```python
from build123d import *

# Parameters (mm, degrees)
F0_R     = 7.5
F0_R_2   = 6.1
F1_DEPTH = 40
F2_R     = 1.6
F3_DEPTH = 1


with BuildPart() as f1:
    # F0 (on Front) → F1 (new body)
    with BuildSketch(Plane.XZ):
        Circle(F0_R)
        Circle(F0_R_2, mode=Mode.SUBTRACT)
    extrude(amount=F1_DEPTH)

    # F2 (on Top) → F3 (join, symmetric)
    with BuildSketch(Plane.XY):
        Polygon((14.5, 0), (6.5, 0), (6.5, -15.75), (14.5, -7.75), align=None)
        with Locations((11.25, -4.75)):
            Circle(F2_R, mode=Mode.SUBTRACT)
        Polygon((6.5, -24.25), (6.5, -40), (14.5, -40), (14.5, -32.25), align=None)
        with Locations((11.25, -35.25)):
            Circle(F2_R, mode=Mode.SUBTRACT)
        Polygon((-6.5, -33), (-6.5, -7), (-14.5, -18.25), (-14.5, -21.75), align=None)
        with Locations((-11.25, -20)):
            Circle(F2_R, mode=Mode.SUBTRACT)
    extrude(amount=F3_DEPTH, both=True)


solid = f1.part
```
CAD build for the part. Positions are in the model's coordinates, mm. A direction names the side the tool comes from. Round coordinates to 2 decimals unless told otherwise and drop trailing zeros. Loops run counter-clockwise (first coordinate to the right, second up) from the corner with the lowest first, then second, coordinate; pieces in that order, holes last. Notation, with made-up numbers: (80.25, -6.75) - (95.25, -6.75) arc R16 cw to (95.25, -2.75) - close; hole circle Ø9 at (-14, 26.5). An arc over 180 degrees is marked (long way). Return JSON: item names as keys, results as strings. Group by question number.
Q1. Two-plate mould, pull along X, no slides. Class faces 1 (the face through (9.65, -4.68, -0.01)), 2 (the face through (-11.016, -26.649, 0.014)), 3 (the face through (9, -6, -1)), 4 (the face through (14.5, -4, 0)): +X half, -X half, draft (parallel to the pull), parting line (faces both ways), or undercut.
Q2. Band-saw the part on A-A on x = 0. Give the cut face in (y, z).
Q3. Band-saw the part on C-C on z = 0. Give the cut face in (x, y), plus the area to 3 significant figures.
Q4. Flat gauge pins, fed straight in: pin 1 Ø4 at (y, z) = (-29, 4.5) entering from -X; pin 2 Ø3.5 at (x, y) = (9.5, -35.5) entering from +Z; pin 3 Ø8 at (x, y) = (9.5, -30) entering from -Z; pin 4 Ø8 at (x, z) = (2, -2) entering from +Y. Where does each tip first touch, or does it go through?
Q5. Band-saw the part on B-B on y = -35.25. Give the cut face in (x, z), plus the area to 3 significant figures.
Q6. Drill centre lines: line 1 along Z through (x, y) = (0, -16); line 2 along Y through (x, z) = (11.25, -0.1); line 3 along Z through (x, y) = (13.25, -1.5). Where is each one in solid material? Low to high. Write a range as [from, to].
Q7. Band-saw the part on D-D on x = 11.25. Give the cut face in (y, z), plus the area to 3 significant figures.
Q8. Tool access for faces 5 (the face through (9, -34, 1)), 6 (the face through (-9, -20, -1)), 7 (the face through (10.92, -11.33, -0.01)), 8 (the face through (-9, -20, 1)): list every direction of +Z, -Z, +X, -X, +Y, -Y with a clear straight run to the whole face (end or side of a thin tool).
Solutions:
{
 "1": {"face 1": "undercut", "face 2": "-X half", "face 3": "draft", "face 4": "+X half"},
 "2": {"outline": "(-40, -7.5) - (0, -7.5) - (0, -6.1) - (-40, -6.1) - close; (-40, 6.1) - (0, 6.1) - (0, 7.5) - (-40, 7.5) - close"},
 "3": {"outline": "(-14.5, -21.75) - (-7.5, -31.59) - (-7.5, -40) - (-6.1, -40) - (-6.1, 0) - (-7.5, 0) - (-7.5, -8.41) - (-14.5, -18.25) - close; (6.1, -40) - (14.5, -40) - (14.5, -32.25) - (7.5, -25.25) - (7.5, -14.75) - (14.5, -7.75) - (14.5, 0) - (6.1, 0) - close; hole circle Ø3.2 at (-11.25, -20); hole circle Ø3.2 at (11.25, -35.25); hole circle Ø3.2 at (11.25, -4.75)", "area": "339 mm^2"},
 "4": {"pin 1": "stops at x = -7.07", "pin 2": "stops at z = 1", "pin 3": "stops at z = -5.1", "pin 4": "stops at y = 0"},
 "5": {"outline": "(7.43, -1) - (9.65, -1) - (9.65, 1) - (7.43, 1) arc R7.5 ccw (long way) to start; (12.85, -1) - (14.5, -1) - (14.5, 1) - (12.85, 1) - close; hole circle Ø12.2 at (0, 0)", "area": "67.5 mm^2"},
 "6": {"line 1": "z = [-7.5, -6.1], [6.1, 7.5]", "line 2": "y = [-40, -36.85], [-33.65, -29], [-11, -6.35], [-3.15, 0]", "line 3": "z = [-1, 1]"},
 "7": {"outline": "(-40, -1) - (-36.85, -1) - (-36.85, 1) - (-40, 1) - close; (-33.65, -1) - (-29, -1) - (-29, 1) - (-33.65, 1) - close; (-11, -1) - (-6.35, -1) - (-6.35, 1) - (-11, 1) - close; (-3.15, -1) - (0, -1) - (0, 1) - (-3.15, 1) - close", "area": "31.2 mm^2"},
 "8": {"face 5": "+Z, +X, +Y, -Y", "face 6": "-Z, -X, +Y, -Y", "face 7": "+Z, -Z, +X", "face 8": "+Z, -X, +Y, -Y"}
}
